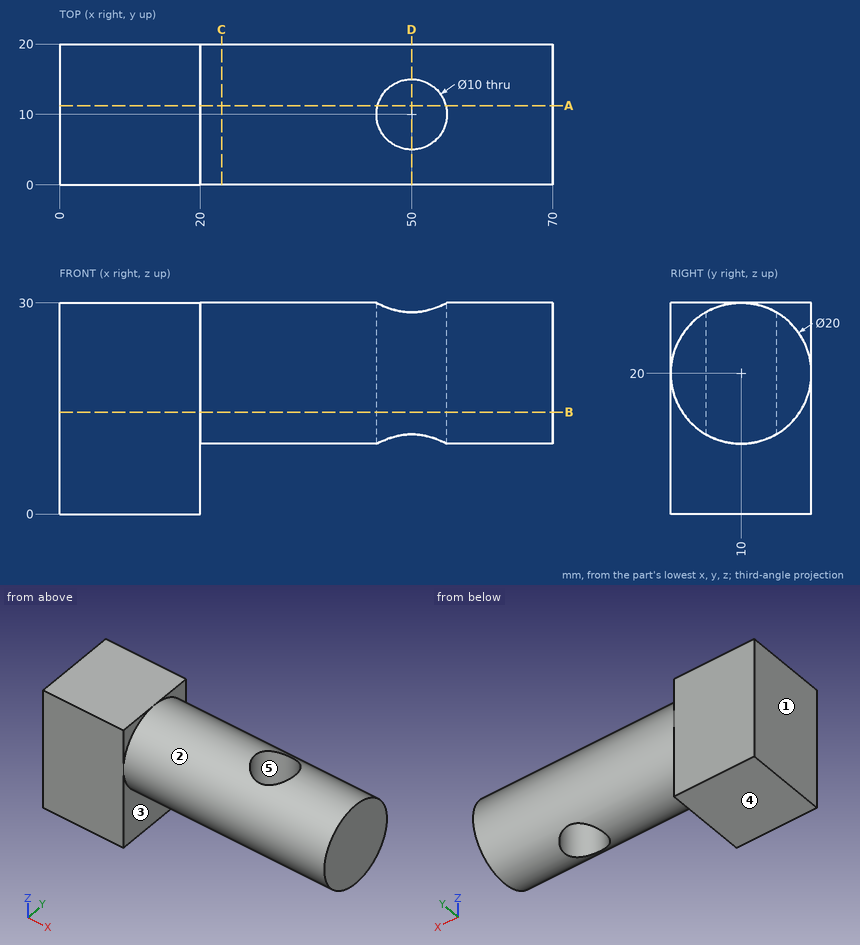
Here's the drawing with two shaded views (mm, measured from the low corner). I have some questions. A direction names the side the tool comes from. Give positions to 0.01 mm unless a question says otherwise; leave off trailing zeros. Write each loop counter-clockwise with the first axis right and the second up, starting at its lowest first coordinate (ties: lowest second). Pieces come first, ordered by that corner, then holes. Notation, with made-up numbers: (27, 39.5) - (58, 39.5) arc R33 cw to (58, 70.5) - close; hole circle Ø7 at (-14.75, -37). An arc over 180 degrees is marked (long way). Write item = value, one per line. Start each with the question number.
1. Imagine slicing it at C-C (x = 23). Please give me the cut outline in (y, z).
2. Thinking about a two-plate mould opening in X: for the marked faces 3, 4 and 5, which applies, released by +X, released by -X, zero draft, split by the parting line, or undercut?
3. On a 3-axis mill with a long thin cutter (end or side, diameter ignored), from which of +Z, -Z, +X, -X, +Y, -Y can I reach the whole of each face in a straight line? I mean the marked faces 1 and 2. Say none if no direction works.
4. Please list where these lines run through material, in increasing order: line 1 (X direction, y = 12.75, z = 7.5); line 2 (Y direction, x = 50, z = 24); line 3 (Z direction, x = 58, y = 10).
5. Imagine slicing it at D-D (x = 50). Please give me the cut outline in (y, z).
6. Imagine slicing it at A-A (y = 11.25). Please give me the cut outline in (x, z).
7. For pin 1 (6 mm diameter, centred on x = 60.5, y = 13.5, fed in from +Z); pin 2 (4 mm diameter, centred on x = 47, y = 4, fed in from -Z); pin 3 (3 mm diameter, centred on x = 28.5, y = 5, fed in from +Z); pin 4 (8 mm diameter, centred on x = 50, y = 10, fed in from +Z), each with a flat end and sliding along its axis, tell me the tip position at first contact or that it passes through.
8. Imagine slicing it at B-B (z = 14.5). Please give me the cut outline in (x, y), and give its area (3 significant figures).
Worked answers:
q1.outline = circle Ø20 at (10, 20)
q2.face_3 = released by +X
q2.face_4 = zero draft
q2.face_5 = undercut
q3.face_1 = +Z, -Z, -X, +Y, -Y
q3.face_2 = +X
q4.line_1 = 0 to 20
q4.line_2 = 0.83 to 5, 15 to 19.17
q4.line_3 = 10 to 30
q5.outline = (5, 11.34) - (5, 28.66) arc R10 ccw to start; (15, 11.34) arc R10 ccw to (15, 28.66) - close
q6.outline = (0, 0) - (20, 0) - (20, 10.08) - (45.16, 10.08) - (45.16, 29.92) - (20, 29.92) - (20, 30) - (0, 30) - close; (54.84, 10.08) - (70, 10.08) - (70, 29.92) - (54.84, 29.92) - close
q7.pin_1 = 29.99
q7.pin_2 = 10.83
q7.pin_3 = 29.37
q7.pin_4 = through
q8.outline = (0, 0) - (20, 0) - (20, 1.65) - (70, 1.65) - (70, 18.35) - (20, 18.35) - (20, 20) - (0, 20) - close; hole circle Ø10 at (50, 10)
q8.area = 1,160 mm2
